Input: dimensioned drawing with shaded views. Units: mm. Origin: part minimum x, y, z. A direction names the side the tool comes from. Round coordinates to 2 decimals unless told otherwise and drop trailing zeros. Loops run counter-clockwise (first coordinate to the right, second up) from the corner with the lowest first, then second, coordinate; pieces in that order, holes last. Notation, with made-up numbers: (-7.5, -20) - (25.5, -20) arc R25 cw to (25.5, 10) - close; hole circle Ø2 at (1, -29). An arc over 180 degrees is marked (long way). One line per question, with ' | ' between items.
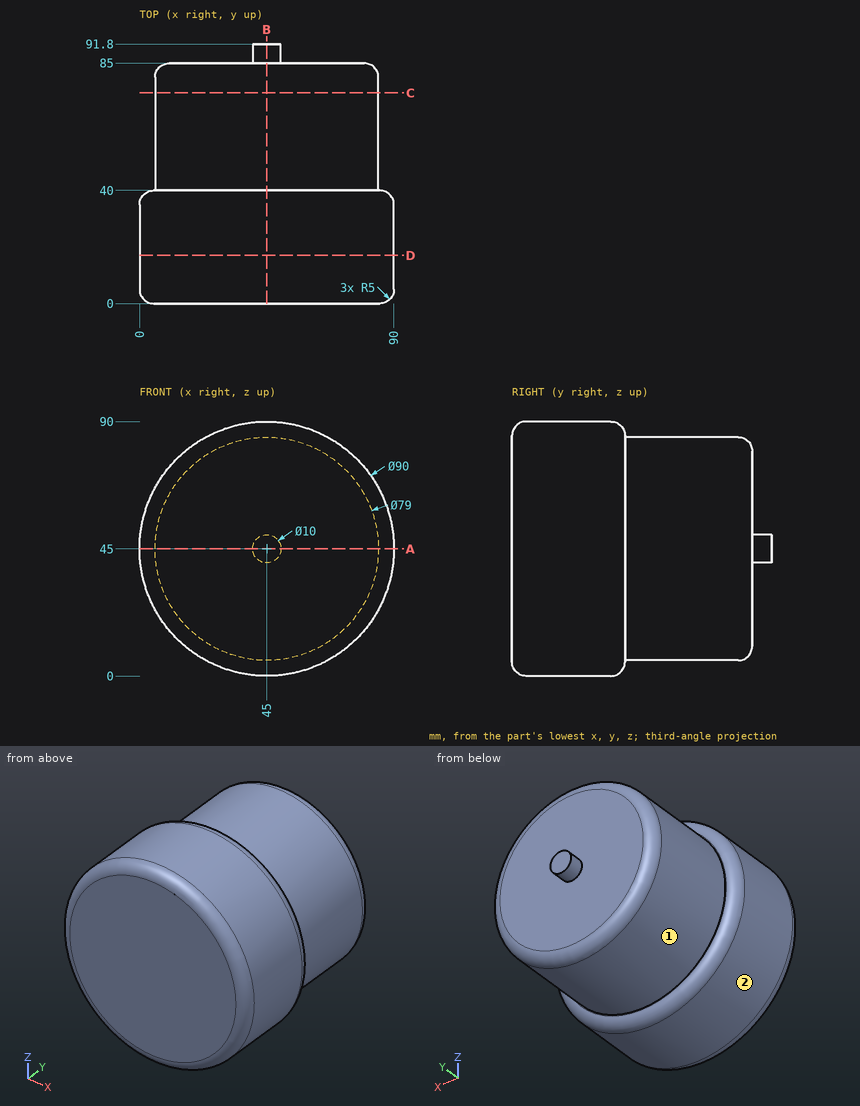
1. Access query for the marked faces 1 and 2. Directions: +Z, -Z, +X, -X, +Y, -Y. A direction counts if a zero-diameter tool reaches every point of the face in a straight line with its end or side. Return the directions, or none.
Worked out:
face 1: +Y | face 2: +Y, -Y
2. Section query D-D, the plane y = 17. Return loops of the section in (x, z).
Worked out:
outline: circle Ø90 at (45, 45)
3. Section query C-C, the plane y = 74.5. Return loops of the section in (x, z), plus the area to 3 significant figures.
Worked out:
outline: circle Ø79 at (45, 45) | area: 4,900 mm2
4. Section query B-B, the plane x = 45. Return loops of the section in (y, z).
Worked out:
outline: (0, 5) arc R5 ccw to (5, 0) - (35, 0) arc R5 ccw to (40, 5) - (40, 5.5) - (80, 5.5) arc R5 ccw to (85, 10.5) - (85, 40) - (91.8, 40) - (91.8, 50) - (85, 50) - (85, 79.5) arc R5 ccw to (80, 84.5) - (40, 84.5) - (40, 85) arc R5 ccw to (35, 90) - (5, 90) arc R5 ccw to (0, 85) - close
5. Section query A-A, the plane z = 45. Return loops of the section in (x, y).
Worked out:
outline: (0, 5) arc R5 ccw to (5, 0) - (85, 0) arc R5 ccw to (90, 5) - (90, 35) arc R5 ccw to (85, 40) - (84.5, 40) - (84.5, 80) arc R5 ccw to (79.5, 85) - (50, 85) - (50, 91.8) - (40, 91.8) - (40, 85) - (10.5, 85) arc R5 ccw to (5.5, 80) - (5.5, 40) - (5, 40) arc R5 ccw to (0, 35) - close
6. Material intervals for probe 1 along Y at (x, z) = (17, 26); probe 2 along Z at (x, y) = (23.5, 8.5); probe 3 along Y at (x, z) = (9, 63), sorted ascending.
Worked out:
probe 1: y = 0 to 85 | probe 2: z = 5.47 to 84.53 | probe 3: y = 0.01 to 39.99
7. Contact query for flat-ended pins moving along their axis: P1, Ø1.5, axis at x = 55.5, y = 79.5, coming from the +Z side; P2, Ø5, axis at x = 15, y = 54, coming from the +Z side; P3, Ø1, axis at x = 30.5, y = 11, coming from the -Z side. Output: stop coordinate, or through.
Worked out:
P1: stops at z = 83.28 | P2: stops at z = 73.35 | P3: stops at z = 2.23
